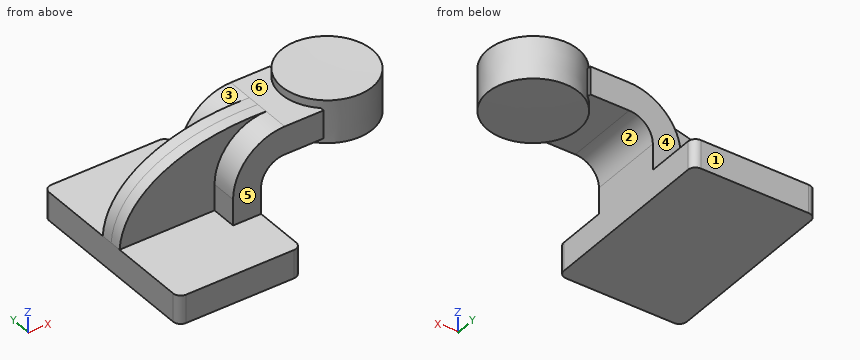
```python
from build123d import *

# Parameters (mm, degrees)
F1_DEPTH = 63.5
F2_DEPTH = 25.4
F3_DEPTH = 7.9375
F5_R     = 5.08


with BuildPart() as f1:
    # F0 (on Front) → F1 (new body, symmetric)
    with BuildSketch(Plane.XZ):
        Polygon((29.4945527817, 9.525), (-34.2594462869, 9.525), (-34.2594462869, -9.525), (48.2905537131, -9.525), (48.2905537131, 9.525), align=None)
    extrude(amount=F1_DEPTH, both=True)

    # F0 (on Front) → F2 (join, symmetric)
    with BuildSketch(Plane.XZ):
        with BuildLine():
            Line((29.4945527817, 27.0002), (29.4945527817, 9.525))
            Line((29.4945527817, 9.525), (48.2905537131, 9.525))
            Line((48.2905537131, 9.525), (48.2905537131, 27.0002))
            ThreePointArc((48.2905537131, 27.0002), (52.9402335618, 38.2255201513), (64.1655537131, 42.8752))
            Line((64.1655537131, 42.8752), (90.2585908771, 42.8752))
            Line((90.2585908771, 42.8752), (90.2585908771, 61.6712009314))
            Line((90.2585908771, 61.6712009314), (64.1655537131, 61.6712009314))
            ThreePointArc((64.1655537131, 61.6712009314), (39.649453844, 51.5162998691), (29.4945527817, 27.0002))
        make_face()
    extrude(amount=F2_DEPTH, both=True)

    # F0 (on Front) → F3 (join, symmetric)
    with BuildSketch(Plane.XZ):
        with BuildLine():
            add(Edge.make_bspline(
                [(-34.2594462869, 9.525), (-32.0006241091, 42.9277569056), (6.9947489537, 64.2252266407), (64.1655537131, 61.6712009314)],
                knots=[0, 0, 0, 0, 111.3853980402, 111.3853980402, 111.3853980402, 111.3853980402], degree=3))
            Line((-34.2594462869, 9.525), (29.4945527817, 9.525))
            Line((29.4945527817, 9.525), (29.4945527817, 27.0002))
            ThreePointArc((29.4945527817, 27.0002), (39.649453844, 51.5162998691), (64.1655537131, 61.6712009314))
        make_face()
    extrude(amount=F3_DEPTH, both=True)

    # F0 (on Front) → F4 (revolve)
    with BuildSketch(Plane.XZ):
        Polygon((110.6271635748, 66.675), (110.6018233776, 61.6712009314), (110.4824542999, 38.1), (141.0585908771, 38.1), (141.0585908771, 66.675), align=None)
    revolve(axis=Axis((110.5548089374, 0, 52.3875), (0.0050641267, 0, 0.9999871772)))

    # F5
    f5_edges = [f1.edges().sort_by_distance(p)[0] for p in [
        (48.290554, 63.5, 0),
        (48.290554, -63.5, 0),
        (-34.259446, -63.5, 0),
        (-34.259446, 63.5, 0),
    ]]
    fillet(f5_edges, radius=F5_R)


solid = f1.part
```
Check sheet for the modelled part. Datum: model origin and axes. Units: mm. Face numbers are marked on the shaded views. A direction names the side the tool comes from. Round coordinates to 2 decimals unless told otherwise and drop trailing zeros. Order: outer loops, then holes, each group sorted by start corner. A loop starts at its lowest first (then second) coordinate and runs counter-clockwise, first axis right, second up. Notation, with made-up numbers: (15.5, 4.25) - (70.5, 4.25) arc R29 cw to (70.5, 32.25) - close; hole circle Ø11 at (80, 77). An arc over 180 degrees is marked (long way). Answer as CSV lines item,"result". Start each with the question number.
1) Draft check along X on the marked faces 1, 2 and 3. Enter one of: +X half, -X half, draft (parallel to the pull), parting line (faces both ways), or undercut.
2) Depth check by flat-ended pin: pin 1 (12 mm diameter, centred on x = 7, z = 40.5, fed in from -Y); pin 2 (8.5 mm diameter, centred on y = -16.5, z = 22, fed in from -X); pin 3 (11 mm diameter, centred on y = 1.5, z = 14, fed in from +X). Enter the tip coordinate at first touch or a pass-through.
3) Scan lines: probe 1 along Z at (x, y) = (80.5, -11); probe 2 along Z at (x, y) = (-19, -17) (3 decimals); probe 3 along Y at (x, z) = (-1.5, 13.5). Record each from-to range of solid material in increasing order.
4) Section check A-A (y = -32.5). Record the cut outline in (x, z) (3 decimals), then the cut area to 3 significant figures.
5) Tool access check on the marked faces 4, 5 and 6. Record the directions out of +Z, -Z, +X, -X, +Y, -Y that give a thin tool (end or side, any length) a straight path to the whole face; none if there is none.
Determined:
1,face 1,"draft"
1,face 2,"undercut"
1,face 3,"-X half"
2,pin 1,"y = -7.94"
2,pin 2,"x = 29.49"
2,pin 3,"x = 48.29"
3,probe 1,"42.88 to 61.67"
3,probe 2,"-9.525 to 9.525"
3,probe 3,"-7.94 to 7.94"
4,outline,"(-34.259, -9.525) - (48.291, -9.525) - (48.291, 9.525) - (-34.259, 9.525) - close"
4,area,"1,570 mm^2"
5,face 4,"+Z, -X, +Y"
5,face 5,"+Z, -X, -Y"
5,face 6,"+Z"
